CAD build for the part. Positions are in the model's coordinates, mm. A direction names the side the tool comes from. Coordinates: 2 decimals unless noted, no trailing zeros. Loops run counter-clockwise (first coordinate to the right, second up) from the corner with the lowest first, then second, coordinate; pieces in that order, holes last.
1) Which spindle directions (+Z, -Z, +X, -X, +Y, -Y) get a long thin tool onto all of the face, cutting with end or side? Do faces 4 (the flat face through (0, -16, 14)), 5 (the flat face through (23.5, -9.2, 14.4)). Say none if no direction does.
2) Saw through at C-C, the plane x = 1.5. Write the cut outline in (y, z).
3) Two-plate mould, pull along Z, no slides. Class faces 1 (the cylindrical face through (22.54, 1.48, -3)), 2 (the flat face through (0, -14, 17)), 3 (the flat face through (0, 0, 1)): +Z half, -Z half, draft (parallel to the pull), parting line (faces both ways), or undercut.
4) Saw through at A-A, the plane x = -7. Write the cut outline in (y, z), and give its area (3 significant figures).
5) Pin check, flat tips, straight feed: pin 1 Ø9.5 at (x, y) = (6.5, -13.5) entering from -Z; pin 2 Ø8 at (x, z) = (6.5, -3) entering from -Y. Stop position of each tip, or through.
6) Wall check: line 1 along X through (y, z) = (2.1, 0); line 2 along Z through (x, y) = (-13, 1); line 3 along Z through (x, y) = (16, -7.5). Give the ranges that are in metal, low to high.
7) Saw through at D-D, the plane z = 9.25. Write the cut outline in (x, y), and give its area (3 significant figures).
8) Saw through at B-B, the plane z = 0. Write the cut outline in (x, y).
```python
from build123d import *

# Parameters (mm, degrees)
SKETCH1_W           = 47
SKETCH1_H           = 24
SKETCH1_R           = 10
BOSS_EXTRUDE1_DEPTH = 3
SKETCH2_W           = 47
SKETCH2_H           = 2
BOSS_EXTRUDE2_DEPTH = 3
SKETCH3_W           = 47
SKETCH3_H           = 3
BOSS_EXTRUDE6_DEPTH = 35


with BuildPart() as part:
    # Sketch1 → Boss-Extrude1 (new body)
    with BuildSketch(Plane(origin=(0, 0, 0), x_dir=(1, 0, 0), z_dir=(0, 1, 0))):
        Rectangle(SKETCH1_W, SKETCH1_H)
        with Locations((-13, 0)):
            Circle(SKETCH1_R, mode=Mode.SUBTRACT)
        with Locations((13, 0)):
            Circle(SKETCH1_R, mode=Mode.SUBTRACT)
    extrude(amount=BOSS_EXTRUDE1_DEPTH)

    # Sketch2 → Boss-Extrude2 (add)
    with BuildSketch(Plane(origin=(0, 3, 0), x_dir=(1, 0, 0), z_dir=(0, 1, 0))):
        with Locations((0, -13)):
            Rectangle(SKETCH2_W, SKETCH2_H)
    extrude(amount=-BOSS_EXTRUDE2_DEPTH)

    # Sketch3 → Boss-Extrude6 (add)
    with BuildSketch(Plane(origin=(0, 3, 0), x_dir=(1, 0, 0), z_dir=(0, 1, 0))):
        with Locations((0, -15.5)):
            Rectangle(SKETCH3_W, SKETCH3_H)
    extrude(amount=-BOSS_EXTRUDE6_DEPTH)


solid = part.part
```
Data:
1. face 4: -Z, +X, -X, -Y
1. face 5: +Z, -Z, +X, +Y, -Y
2. outline: (-32, 14) - (0, 14) - (0, -12) - (3, -12) - (3, 17) - (-32, 17) - close
3. face 1: undercut
3. face 2: +Z half
3. face 3: draft
4. outline: (-32, 14) - (0, 14) - (0, 8) - (3, 8) - (3, 17) - (-32, 17) - close; (0, -12) - (3, -12) - (3, -8) - (0, -8) - close
4. area: 135 mm2
5. pin 1: stops at z = 14
5. pin 2: stops at y = 0
6. line 1: x = -23.5 to -23, -3 to 3, 23 to 23.5
6. line 2: z = -12 to -10, 10 to 17
6. line 3: z = 14 to 17
7. outline: (-23.5, 0) - (-16.8, 0) - (-16.8, 3) - (-23.5, 3) - close; (-9.2, 0) - (9.2, 0) - (9.2, 3) - (-9.2, 3) - close; (16.8, 0) - (23.5, 0) - (23.5, 3) - (16.8, 3) - close
7. area: 95.4 mm2
8. outline: (-23.5, 0) - (-23, 0) - (-23, 3) - (-23.5, 3) - close; (-3, 0) - (3, 0) - (3, 3) - (-3, 3) - close; (23, 0) - (23.5, 0) - (23.5, 3) - (23, 3) - close
